Autodesk Inventor part; units mm, degrees
ref_plane "YZ Plane" through (0, 0, 0) normal (1, 0, 0) x (0, 1, 0)
ref_plane "XZ Plane" through (0, 0, 0) normal (0, 1, 0) x (-1, 0, 0)
ref_plane "XY Plane" through (0, 0, 0) normal (0, 0, 1) x (1, 0, 0)
sketch "Sketch1" plane through (0, 0, 0) normal (0, 0, 1) x (1, 0, 0)
  circle A0 centre (0, 0) radius 6.5484
  circle A1 centre (0, 0) radius 10.3188
  dimension "d0" = 20.6375
  dimension "d1" = 13.0969
extrude "Extrusion1" add sketch "Sketch1" against normal blind 9.525
sketch "Sketch2" plane through (0, 0, -9.525) normal (0, 0, -1) x (-1, 0, 0)
  circle A0 centre (0, 0) radius 6.5484
  circle A1 centre (0, 0) radius 10.3188
  circle A2 centre (0, 0) radius 9.1281
  dimension "d4" = 18.2563
extrude "Extrusion2" add sketch "Sketch2" along normal blind 11.1125 contours A2
sketch "Sketch3" plane through (0, 0, 0) normal (0, 1, 0) x (-1, 0, 0)
  line L0 (-10.3188, 0) -> (10.3188, 0)
  line L1 (-1.1906, 0) -> (-1.1906, -3.175)
  line L2 (-1.1906, -3.175) -> (1.1906, -3.175)
  line L3 (1.1906, -3.175) -> (1.1906, 0)
  point P0 (0, -3.175)
  point P1 (0, 0)
  dimension "d7" = 3.175
  dimension "d8" = 2.3813
extrude "Extrusion3" cut sketch "Sketch3" along normal through all both and the other way through all
thread "Thread1"
properties part number "Collar" material "Steel, Mild"
Work out the finished part from the listing and answer in its coordinate system (mm). A direction names the side the tool comes from. Give positions to 0.01 mm unless a question says otherwise; leave off trailing zeros. Write each loop counter-clockwise with the first axis right and the second up, starting at its lowest first coordinate (ties: lowest second). Pieces come first, ordered by that corner, then holes.
Q1. The part is cut by section A-A on y = 0. Give the vertices of the cut face in (x, z) (1 decimal), and give its area (3 significant figures).
Answer:
outline: (-10.3, -9.5) - (-9.1, -9.5) - (-9.1, -20.6) - (-6.5, -20.6) - (-6.5, 0) - (-10.3, 0) - close; (6.5, -20.6) - (9.1, -20.6) - (9.1, -9.5) - (10.3, -9.5) - (10.3, 0) - (6.5, 0) - close
area: 129 mm2
Q2. Given pin 1 (12 mm diameter, centred on x = 0, y = 0, fed in from +Z); pin 2 (0.7 mm diameter, centred on x = -0.5, y = 7.5, fed in from +Z) (3 decimals); pin 3 (1.6 mm diameter, centred on y = -7.5, z = -1.5, fed in from -X); pin 4 (1.5 mm diameter, centred on x = -0.5, z = -15.5, fed in from -Y), each flat-ended and moving along its own axis, determine where each tip first touches the part or whether it passes through.
Answer:
pin 1: passes through
pin 2: stops at z = -3.175
pin 3: stops at x = -7.85
pin 4: stops at y = -9.13
Q3. For a pull along X with two mould halves and no side action, classify faces 1 (the face through (1.191, -8, -2)), 2 (the face through (-6, -4, -20.638)), 3 (the face through (-8.707, -2.742, -15.003)) as released by +X, released by -X, zero draft, split by the parting line, or undercut.
Answer:
face 1: undercut
face 2: zero draft
face 3: split by the parting line
Q4. The part is cut by section D-D on y = 7.5. Give the vertices of the cut face in (x, z) (1 decimal).
Answer:
outline: (-7.1, -9.5) - (-5.2, -9.5) - (-5.2, -20.6) - (5.2, -20.6) - (5.2, -9.5) - (7.1, -9.5) - (7.1, 0) - (1.2, 0) - (1.2, -3.2) - (-1.2, -3.2) - (-1.2, 0) - (-7.1, 0) - close
Q5. A tool of negligible diameter and unlimited length cuts with its end or side. For faces 4 (the face through (-7, 0, 0)), 5 (the face through (2.2, -9.1, -9.525)), 6 (the face through (0, 8, -3.175)), from which of +Z, -Z, +X, -X, +Y, -Y can it reach the whole face along a straight path? Write none if from no direction.
Answer:
face 4: +Z, +X, -X, +Y, -Y
face 5: -Z
face 6: +Z, +Y, -Y
Q6. The part is cut by section B-B on x = -3.75. Give the vertices of the cut face in (y, z) (1 decimal), and give its area (3 significant figures).
Answer:
outline: (-9.6, -9.5) - (-8.3, -9.5) - (-8.3, -20.6) - (-5.4, -20.6) - (-5.4, 0) - (-9.6, 0) - close; (5.4, -20.6) - (8.3, -20.6) - (8.3, -9.5) - (9.6, -9.5) - (9.6, 0) - (5.4, 0) - close
area: 147 mm2
Q7. The part is cut by section C-C on z = -7.5. Give the vertices of the cut face in (x, y), and give its area (3 significant figures).
Answer:
outline: circle Ø20.64 at (0, 0); hole circle Ø13.1 at (0, 0)
area: 200 mm2
Q8. Straight lines are drawn through the part: L1, parallel to X at y = 0, z = -6; L2, parallel to Y at x = 0.75, z = -18.75. For each, find the intervals that lie inside material, in ascending order.
Answer:
L1: x = -10.32 to -6.55, 6.55 to 10.32
L2: y = -9.1 to -6.51, 6.51 to 9.1
